```python
from build123d import *

# Parameters (mm, degrees)
F0_R     = 1
F1_DEPTH = 25


with BuildPart() as f1:
    # F0 (on Top) → F1 (new body)
    with BuildSketch(Plane.XY):
        with BuildLine():
            ThreePointArc((1.05758, -1.394283), (1.567365, -0.778375), (1.75, 0))
            ThreePointArc((1.75, 0), (0.96819, 1.457775), (-0.678694, 1.613033))
            ThreePointArc((-0.678694, 1.613033), (-1.515544, -0.875), (1.05758, -1.394283))
        make_face()
        Circle(F0_R, mode=Mode.SUBTRACT)
        with BuildLine():
            ThreePointArc((-0.678694, 1.613033), (0.96819, 1.457775), (1.75, 0))
            ThreePointArc((1.75, 0), (1.567365, -0.778375), (1.05758, -1.394283))
            Line((1.05758, -1.394283), (2.895761, 0))
            Line((2.895761, 0), (5.800484, 2.203267))
            ThreePointArc((5.800484, 2.203267), (4.330127, 2.5), (4.808327, 3.921733))
            Line((4.808327, 3.921733), (-0.678694, 1.613033))
        make_face()
    extrude(amount=F1_DEPTH)


solid = f1.part
```
Work out the finished part from the listing and answer in its coordinate system (mm). Coordinates: 2 decimals unless noted, no trailing zeros. Write each loop counter-clockwise with the first axis right and the second up, starting at its lowest first coordinate (ties: lowest second). Pieces come first, ordered by that corner, then holes.
Q1. Determine the mould class of faces 1 (the face through (-1.536, -0.839, 12.325)), 2 (the face through (2.103, 2.784, 12.325)), 3 (the face through (0, -1, 12)) for opening direction X: released by +X, released by -X, zero draft, split by the parting line, or undercut.
Q2. Find the intervals of material crossed by line 1 (X direction, y = 0.3, z = 14.5); line 2 (Y direction, x = 0, z = 9.5); line 3 (Y direction, x = 0.75, z = 15.75), in increasing order.
Q3. A cutting plane is placed at B-B, the plane x = 0. Give the vertices of the cut face in (y, z), then the cut area to 3 significant figures.
Q4. A cutting plane is placed at A-A, the plane y = -0.4. Give the vertices of the cut face in (x, z), then the cut area to 3 significant figures.
Q5. A cutting plane is placed at C-C, the plane y = 3. Give the vertices of the cut face in (x, z), then the cut area to 3 significant figures.
Q6. Each of these flat-tipped pins is pushed along its axis until it touches: pin 1 Ø2.5 at (x, y) = (5.2, 3) entering from +Z; pin 2 Ø2 at (y, z) = (0.5, 17.5) entering from +X. Where does it stop, or does it pass through?
Q7. A cutting plane is placed at D-D, the plane x = 2. Give the vertices of the cut face in (y, z).
Findings below:
1. face 1: split by the parting line
1. face 2: released by -X
1. face 3: undercut
2. line 1: x = -1.72 to -0.95, 0.95 to 3.29
2. line 2: y = -1.75 to -1, 1 to 1.9
2. line 3: y = -1.58 to -0.66, 0.66 to 2.21
3. outline: (-1.75, 0) - (-1, 0) - (-1, 25) - (-1.75, 25) - close; (1, 0) - (1.9, 0) - (1.9, 25) - (1, 25) - close
3. area: 41.2 mm2
4. outline: (-1.7, 0) - (-0.92, 0) - (-0.92, 25) - (-1.7, 25) - close; (0.92, 0) - (2.37, 0) - (2.37, 25) - (0.92, 25) - close
4. area: 56.0 mm2
5. outline: (2.62, 0) - (4.2, 0) - (4.2, 25) - (2.62, 25) - close
5. area: 39.5 mm2
6. pin 1: stops at z = 25
6. pin 2: stops at x = 4.87
7. outline: (-0.68, 0) - (2.74, 0) - (2.74, 25) - (-0.68, 25) - close
